The listing builds one solid part. Answer for the finished solid, in the listing's coordinates (mm). A direction names the side the tool comes from. Round coordinates to 2 decimals unless told otherwise and drop trailing zeros. Order: outer loops, then holes, each group sorted by start corner. A loop starts at its lowest first (then second) coordinate and runs counter-clockwise, first axis right, second up. Notation, with made-up numbers: (49.25, -6) - (80.25, -6) arc R23 cw to (80.25, 5) - close; hole circle Ø7 at (41.5, 14). An arc over 180 degrees is marked (long way). Use CSV: the item, a comma, the result in double quotes. Start each with the question number.
Item 1: For faces 1 (the flat face through (-2, 14.738, 0)), 2 (the cylindrical face through (1.617, 18.589, 0.67)), 3 (the flat face through (-2, 20, 0)), determine the directions among +Z, -Z, +X, -X, +Y, -Y from which every point of the face is accessible in a straight line to the end or side of a thin tool.
Item 2: Straight lines are drawn through the part: line 1 along X through (y, z) = (16.75, -1.75); line 2 along X through (y, z) = (13.25, 0); line 3 along Y through (x, z) = (-2.5, 1.75). For each, find the intervals that lie inside material, in ascending order. Write a range as [from, to].
Item 3: Find section C-C, the plane z = 0. Give the vertices of the cut face in (x, y), plus the area to 3 significant figures.
Item 4: Find section A-A, the plane x = 0. Give the vertices of the cut face in (y, z), plus the area to 3 significant figures.
Item 5: Find section D-D, the plane z = -3.25. Give the vertices of the cut face in (x, y).
Item 6: Flat-ended cylindrical pins translate along their axes: P1, Ø2, axis at x = 0, z = 0, coming from the +Y side; P2, Ø2.5, axis at x = 0, y = 5, coming from the -Z side. Find the tip coordinate at first contact, or state that the pin passes through.
Item 7: Determine the mould class of faces 4 (the flat face through (0, 7, 0)), 5 (the flat face through (0, 0, 0)), 6 (the flat face through (4.5, 10, 0)) for opening direction X: +X half, -X half, draft (parallel to the pull), parting line (faces both ways), or undercut.
Item 8: Find section B-B, the plane y = 5. Give the vertices of the cut face in (x, z), plus the area to 3 significant figures.
```python
from build123d import *

# Parameters (mm, degrees)
SKETCH1_W           = 9
SKETCH1_H           = 12.5
BOSS_EXTRUDE1_DEPTH = 20
SKETCH2_R           = 1
CUT_EXTRUDE1_DEPTH  = 13.5
SKETCH3_W           = 5.32
SKETCH3_H           = 2.4
CUT_EXTRUDE2_DEPTH  = 13.5
SKETCH4_R           = 1.75
CUT_EXTRUDE3_DEPTH  = 13


with BuildPart() as part:
    # Sketch1 → Boss-Extrude1 (new body)
    with BuildSketch(Plane(origin=(0, 0, 0), x_dir=(1, 0, 0), z_dir=(0, 1, 0))):
        Rectangle(SKETCH1_W, SKETCH1_H)
    extrude(amount=BOSS_EXTRUDE1_DEPTH)

    # Sketch2 → Cut-Extrude1 (cut, through all)
    with BuildSketch(Plane.XY.offset(6.25)):
        with Locations((0, 5)):
            Circle(SKETCH2_R)
    extrude(amount=-CUT_EXTRUDE1_DEPTH, mode=Mode.SUBTRACT)

    # Sketch3 → Cut-Extrude2 (cut, through all)
    with BuildSketch(Plane.XY.offset(6.25)):
        with Locations((0, 15.93763485)):
            Rectangle(SKETCH3_W, SKETCH3_H)
    extrude(amount=-CUT_EXTRUDE2_DEPTH, mode=Mode.SUBTRACT)

    # Sketch4 → Cut-Extrude3 (cut)
    with BuildSketch(Plane(origin=(0, 20, 0), x_dir=(1, 0, 0), z_dir=(0, 1, 0))):
        Circle(SKETCH4_R)
    extrude(amount=-CUT_EXTRUDE3_DEPTH, mode=Mode.SUBTRACT)


solid = part.part
```
Worked out:
1,face 1,"+Z, -Z"
1,face 2,"+Y"
1,face 3,"+Z, -Z, +X, -X, +Y"
2,line 1,"x = [-4.5, -2.66], [2.66, 4.5]"
2,line 2,"x = [-4.5, -1.75], [1.75, 4.5]"
2,line 3,"y = [0, 14.74], [17.14, 20]"
3,outline,"(-4.5, 0) - (4.5, 0) - (4.5, 20) - (1.75, 20) - (1.75, 17.14) - (2.66, 17.14) - (2.66, 14.74) - (1.75, 14.74) - (1.75, 7) - (-1.75, 7) - (-1.75, 14.74) - (-2.66, 14.74) - (-2.66, 17.14) - (-1.75, 17.14) - (-1.75, 20) - (-4.5, 20) - close; hole circle Ø2 at (0, 5)"
3,area,"127 mm²"
4,outline,"(0, -6.25) - (4, -6.25) - (4, 6.25) - (0, 6.25) - close; (6, -6.25) - (14.74, -6.25) - (14.74, -1.75) - (7, -1.75) - (7, 1.75) - (14.74, 1.75) - (14.74, 6.25) - (6, 6.25) - close; (17.14, -6.25) - (20, -6.25) - (20, -1.75) - (17.14, -1.75) - close; (17.14, 1.75) - (20, 1.75) - (20, 6.25) - (17.14, 6.25) - close"
4,area,"158 mm²"
5,outline,"(-4.5, 0) - (4.5, 0) - (4.5, 20) - (-4.5, 20) - close; hole (-2.66, 14.74) - (2.66, 14.74) - (2.66, 17.14) - (-2.66, 17.14) - close; hole circle Ø2 at (0, 5)"
6,P1,"stops at y = 7"
6,P2,"stops at z = -6.25"
7,face 4,"undercut"
7,face 5,"draft"
7,face 6,"+X half"
8,outline,"(-4.5, -6.25) - (-1, -6.25) - (-1, 6.25) - (-4.5, 6.25) - close; (1, -6.25) - (4.5, -6.25) - (4.5, 6.25) - (1, 6.25) - close"
8,area,"87.5 mm²"
